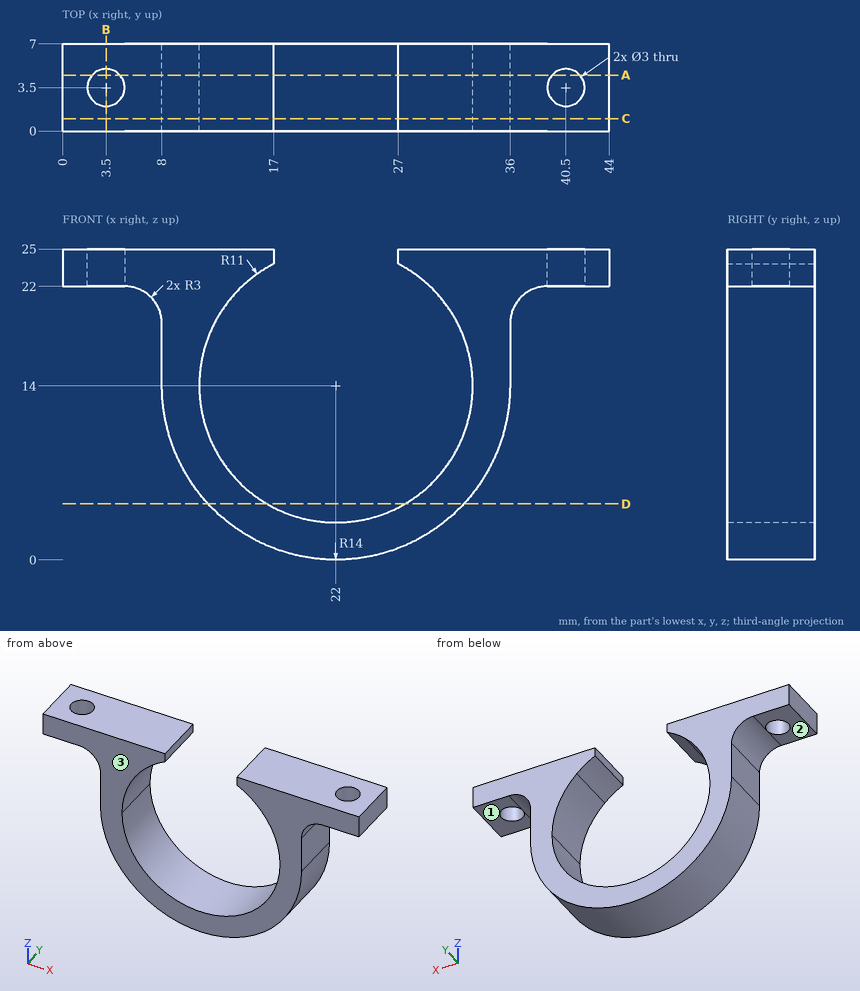
Study the drawing (mm; zero at the part's minimum x, y, z) and answer. A direction names the side the tool comes from. Coordinates: 2 decimals unless noted, no trailing zeros. Order: outer loops, then holes, each group sorted by start corner. A loop starts at its lowest first (then second) coordinate and runs counter-clockwise, first axis right, second up. Notation, with made-up numbers: M 71.5,28 L 94.5,28 A13 cw 94.5,34 Z; hole C 56.25,-24 d2. An arc over 180 degrees is marked long. Answer as a JSON object with one key per item and string values. Group by question number.
1. Section A-A on y = 4.5 is taken. Write down the section's boundary in (x, z), then the cut area to 3 significant figures.
2. Section C-C on y = 1 is taken. Write down the section's boundary in (x, z).
3. Section D-D on z = 4.5 is taken. Write down the section's boundary in (x, y), then the cut area to 3 significant figures.
4. Flat-ended cylindrical pins translate along their axes: P1, Ø1, axis at y = 2.5, z = 4, coming from the +X side; P2, Ø4, axis at y = 4.5, z = 16.5, coming from the +X side; P3, Ø4, axis at x = 22, y = 5.5, coming from the +Z side. Find the tip coordinate at first contact, or state that the pin passes through.
5. Section B-B on x = 3.5 is taken. Write down the section's boundary in (y, z), then the cut area to 3 significant figures.
6. Straight lines are drawn through the part: line 1 (Y direction, x = 40.5, z = 22.65); line 2 (X direction, y = 3.25, z = 23.75); line 3 (X direction, y = 4.5, z = 23). For each, find the intervals that lie inside material, in ascending order.
7. A tool of negligible diameter and unlimited length cuts with its end or side. For the marked faces 1, 2 and 3, from which of +Z, -Z, +X, -X, +Y, -Y can it reach the whole face along a straight path? Write none if from no direction.
Values follow:
{
 "1": {"outline": "M 0,22 L 2.38,22 L 2.38,25 L 0,25 Z; M 4.62,22 L 5,22 A3 cw 8,19 L 8,14 A14 ccw 36,14 L 36,19 A3 cw 39,22 L 39.38,22 L 39.38,25 L 27,25 L 27,23.8 A11 cw long 17,23.8 L 17,25 L 4.62,25 Z; M 41.62,22 L 44,22 L 44,25 L 41.62,25 Z", "area": "270 mm2"},
 "2": {"outline": "M 0,22 L 5,22 A3 cw 8,19 L 8,14 A14 ccw 36,14 L 36,19 A3 cw 39,22 L 44,22 L 44,25 L 27,25 L 27,23.8 A11 cw long 17,23.8 L 17,25 L 0,25 Z"},
 "3": {"outline": "M 11.72,0 L 16.45,0 L 16.45,7 L 11.72,7 Z; M 27.55,0 L 32.28,0 L 32.28,7 L 27.55,7 Z", "area": "66.3 mm2"},
 "4": {"P1": "x = 32.28", "P2": "x = 36", "P3": "z = 3.18"},
 "5": {"outline": "M 0,22 L 2,22 L 2,25 L 0,25 Z; M 5,22 L 7,22 L 7,25 L 5,25 Z", "area": "12.0 mm2"},
 "6": {"line 1": "0 to 2, 5 to 7", "line 2": "0 to 2.02, 4.98 to 16.91, 27.09 to 39.02, 41.98 to 44", "line 3": "0 to 2.38, 4.62 to 15.68, 28.32 to 39.38, 41.62 to 44"},
 "7": {"face 1": "-Z, +X, +Y, -Y", "face 2": "-Z, -X, +Y, -Y", "face 3": "+Z, -Z, +X, -X, -Y"}
}
